```python
from build123d import *

# Parameters (mm, degrees)
SKETCH_1_R               = 49
EXTRUDE_1_DEPTH          = 30
SKETCH_16_R              = 250
SKETCH_16_5_R            = 250
SKETCH_14_OUTSIDE_W      = 643.93
SKETCH_14_OUTSIDE_H      = 643.93
CUT_EXTRUDE_1_DEPTH      = 355.823900134
CUT_EXTRUDE_1_DEPTH_BACK = 355.823900134
SHELL_1_T                = 2
SKETCH_15_OUTSIDE_W      = 604.606
SKETCH_15_OUTSIDE_H      = 202.606
CUT_EXTRUDE_2_DEPTH      = 257.517055963
CUT_EXTRUDE_2_DEPTH_BACK = 257.517055963


with BuildPart() as part:
    # 草图1 → 凸台-拉伸1 (new, symmetric)
    with BuildSketch(Plane(origin=(0, 0, 0), x_dir=(1, 0, 0), z_dir=(0, 1, 0))):
        with Locations(Location((0, 0, 0), (0, 0, 270))):
            Circle(SKETCH_1_R)
    extrude(amount=EXTRUDE_1_DEPTH, both=True)

    # 草图16 → section 0 of loft_1
    with BuildSketch(Plane(origin=(0, 0, 0), x_dir=(1, 0, 0), z_dir=(0, 1, 0)), mode=Mode.PRIVATE) as loft_1_s0:
        Circle(SKETCH_16_R)
    # loft up to a face of the part (loft_1)
    loft([loft_1_s0.sketch, Face(Wire([part.edges().sort_by_distance((35.719462744, 30, -33.542808191))[0]]))])

    # 草图16<5> → section 0 of loft_3
    with BuildSketch(Plane(origin=(0, 0, 0), x_dir=(1, 0, 0), z_dir=(0, 1, 0)), mode=Mode.PRIVATE) as loft_3_s0:
        Circle(SKETCH_16_5_R)
    # loft up to a face of the part (loft_3)
    loft([loft_3_s0.sketch, Face(Wire([part.edges().sort_by_distance((-35.719462744, -30, -33.542808191))[0]]))])

    # 草图14 outside → 切除-拉伸1 (cut, two sides)
    with BuildSketch(Plane(origin=(0, 0, 0), x_dir=(1, 0, 0), z_dir=(0, 1, 0))) as cut_extrude_1_sk:
        Rectangle(SKETCH_14_OUTSIDE_W, SKETCH_14_OUTSIDE_H)
        with BuildLine():
            Line((-250, 0), (-9.604, -48.049590883))
            ThreePointArc((-9.604, -48.049590883), (0, -49), (9.604, -48.049590883))
            Line((9.604, -48.049590883), (250, 0))
            Line((250, 0), (9.604, 48.049590883))
            ThreePointArc((9.604, 48.049590883), (1.6e-08, 49), (-9.603999968, 48.049590889))
            Line((-9.603999968, 48.049590889), (-250, 0))
        make_face(mode=Mode.SUBTRACT)
    extrude(amount=CUT_EXTRUDE_1_DEPTH, mode=Mode.SUBTRACT)
    extrude(cut_extrude_1_sk.sketch, amount=-CUT_EXTRUDE_1_DEPTH_BACK, mode=Mode.SUBTRACT)

    # 抽壳1 (no face opened: a closed hollow body)
    add(offset(amount=-SHELL_1_T, mode=Mode.PRIVATE), mode=Mode.SUBTRACT)

    # 草图15 outside → 切除-拉伸2 (cut, two sides)
    with BuildSketch(Plane(origin=(0, 0, 0), x_dir=(1, 0, 0), z_dir=(0, 1, 0))) as cut_extrude_2_sk:
        Rectangle(SKETCH_15_OUTSIDE_W, SKETCH_15_OUTSIDE_H)
        with BuildLine():
            Line((-9.60400022, -48.049590839), (-164.621347882, -17.065214498))
            Line((-164.621347882, -17.065214498), (-164.621347882, 17.065214498))
            Line((-164.621347882, 17.065214498), (-9.604, 48.049590883))
            ThreePointArc((-9.604, 48.049590883), (0, 49), (9.604, 48.049590883))
            Line((9.604, 48.049590883), (165, 16.989530712))
            Line((165, 16.989530712), (165, -16.989530712))
            Line((165, -16.989530712), (9.604, -48.049590883))
            ThreePointArc((9.604, -48.049590883), (-1.12e-07, -49), (-9.60400022, -48.049590839))
        make_face(mode=Mode.SUBTRACT)
    extrude(amount=CUT_EXTRUDE_2_DEPTH, mode=Mode.SUBTRACT)
    extrude(cut_extrude_2_sk.sketch, amount=-CUT_EXTRUDE_2_DEPTH_BACK, mode=Mode.SUBTRACT)


solid = part.part
```
Design review of the part built by this model. Coordinates are the model's own, in mm. A direction names the side the tool comes from. Coordinates: 2 decimals unless noted, no trailing zeros. Loops run counter-clockwise (first coordinate to the right, second up) from the corner with the lowest first, then second, coordinate; pieces in that order, holes last.
Q1. The part is to be moulded in two halves that separate along Y. For faces 3 (the face through (0, 0, 47)), 4 (the face through (-70.7, 0.4, 33.8)), 5 (the face through (85.52, 24.55, 0.55)), 6 (the face through (0, 0, -49)), say which applies: +Y half, -Y half, draft (parallel to the pull), parting line (faces both ways), or undercut.
Reported:
face 3: undercut
face 4: undercut
face 5: +Y half
face 6: draft
Q2. To check wall thickness, follow line 1 (Y direction, x = 35.5, z = 0); line 2 (Z direction, x = 27, y = -20); line 3 (Z direction, x = 110.5, y = -18). State the ranges of each line that lie inside material, in increasing order.
Reported:
line 1: y = -30 to -28, 28 to 30
line 2: z = -44.57 to -42.53, 42.53 to 44.57
line 3: z = -27.88 to -25.84, 25.84 to 27.88
Q3. For pin 1 (6 mm diameter, centred on x = -42.5, y = -20.5, fed in from -Z); pin 2 (4 mm diameter, centred on x = 104, y = 23, fed in from +Z); pin 3 (1 mm diameter, centred on x = -118, y = -8.5, fed in from +Z), all flat-tipped, find the tip position at first contact; note any pin that passes through.
Reported:
pin 1: stops at z = -42.07
pin 2: stops at z = 29.41
pin 3: stops at z = 26.48
Q4. We need section B-B on y = 18. State the section outline as (x, z) points.
Reported:
outline: (-127.04, -24.58) - (-9.6, -48.05) arc R49 ccw to (9.6, -48.05) - (127.04, -24.58) arc R129.4 ccw to (127.04, 24.58) - (9.6, 48.05) arc R49 ccw to (-9.6, 48.05) - (-127.04, 24.58) arc R129.4 ccw to start; hole (-113.05, -25.33) - (-9.21, -46.09) arc R47 ccw to (9.21, -46.09) - (113.05, -25.33) arc R115.85 ccw to (113.05, 25.33) - (9.21, 46.09) arc R47 ccw to (-9.21, 46.09) - (-113.05, 25.33) arc R115.85 ccw to start
Q5. Tool access review of faces 1 (the face through (85.52, -24.55, 0.55)), 2 (the face through (85.36, -22.55, 0.44)): name each direction out of +Z, -Z, +X, -X, +Y, -Y from which nothing blocks a thin tool from reaching the whole face with its end or side.
Reported:
face 1: +X, -Y
face 2: none
Q6. We need section A-A on y = 0.5. State the section outline as (x, z) points.
Reported:
outline: (-164.62, -17.07) - (-9.6, -48.05) arc R49 ccw to (9.6, -48.05) - (165, -16.99) - (165, -14.95) - (9.21, -46.09) arc R47 cw to (-9.21, -46.09) - (-164.62, -15.03) - close; (-164.62, 15.03) - (-9.21, 46.09) arc R47 cw to (9.21, 46.09) - (165, 14.95) - (165, 16.99) - (9.6, 48.05) arc R49 ccw to (-9.6, 48.05) - (-164.62, 17.07) - close
